from build123d import *

# Parameters (mm, degrees)
Y_KSEKLIK_EKSTR_ZYON1_DEPTH = 100


with BuildPart() as part:
    # Çizim1 → Yükseklik-Ekstrüzyon1 (new body)
    with BuildSketch(Plane.XY.offset(100)):
        with BuildLine():
            Line((6, -28.5), (6, -30))
            Line((6, -30), (26, -30))
            ThreePointArc((26, -30), (28.828427125, -28.828427125), (30, -26))
            Line((30, -26), (30, -6))
            Line((30, -6), (28.5, -6))
            Line((28.5, -6), (28.5, -5))
            Line((28.5, -5), (24, -5))
            Line((24, -5), (24, -10))
            Line((24, -10), (20, -10))
            Line((20, -10), (17, -7))
            Line((17, -7), (17, -0.5))
            Line((17, -0.5), (16.5, 0))
            Line((16.5, 0), (17, 0.5))
            Line((17, 0.5), (17, 7))
            Line((17, 7), (20, 10))
            Line((20, 10), (24, 10))
            Line((24, 10), (24, 5))
            Line((24, 5), (28.5, 5))
            Line((28.5, 5), (28.5, 6))
            Line((28.5, 6), (30, 6))
            Line((30, 6), (30, 26))
            ThreePointArc((30, 26), (28.828427125, 28.828427125), (26, 30))
            Line((26, 30), (6, 30))
            Line((6, 30), (6, 28.5))
            Line((6, 28.5), (5, 28.5))
            Line((5, 28.5), (5, 24))
            Line((5, 24), (10, 24))
            Line((10, 24), (10, 20))
            Line((10, 20), (7, 17))
            Line((7, 17), (0.5, 17))
            Line((0.5, 17), (0, 16.5))
            Line((0, 16.5), (-0.5, 17))
            Line((-0.5, 17), (-7, 17))
            Line((-7, 17), (-10, 20))
            Line((-10, 20), (-10, 24))
            Line((-10, 24), (-5, 24))
            Line((-5, 24), (-5, 28.5))
            Line((-5, 28.5), (-6, 28.5))
            Line((-6, 28.5), (-6, 30))
            Line((-6, 30), (-26, 30))
            ThreePointArc((-26, 30), (-28.828427125, 28.828427125), (-30, 26))
            Line((-30, 26), (-30, 6))
            Line((-30, 6), (-28.5, 6))
            Line((-28.5, 6), (-28.5, 5))
            Line((-28.5, 5), (-24, 5))
            Line((-24, 5), (-24, 10))
            Line((-24, 10), (-20, 10))
            Line((-20, 10), (-17, 7))
            Line((-17, 7), (-17, 0.5))
            Line((-17, 0.5), (-16.5, 0))
            Line((-16.5, 0), (-17, -0.5))
            Line((-17, -0.5), (-17, -7))
            Line((-17, -7), (-20, -10))
            Line((-20, -10), (-24, -10))
            Line((-24, -10), (-24, -5))
            Line((-24, -5), (-28.5, -5))
            Line((-28.5, -5), (-28.5, -6))
            Line((-28.5, -6), (-30, -6))
            Line((-30, -6), (-30, -26))
            ThreePointArc((-30, -26), (-28.828427125, -28.828427125), (-26, -30))
            Line((-26, -30), (-6, -30))
            Line((-6, -30), (-6, -28.5))
            Line((-6, -28.5), (-5, -28.5))
            Line((-5, -28.5), (-5, -24))
            Line((-5, -24), (-10, -24))
            Line((-10, -24), (-10, -20))
            Line((-10, -20), (-7, -17))
            Line((-7, -17), (-0.5, -17))
            Line((-0.5, -17), (0, -16.5))
            Line((0, -16.5), (0.5, -17))
            Line((0.5, -17), (7, -17))
            Line((7, -17), (10, -20))
            Line((10, -20), (10, -24))
            Line((10, -24), (5, -24))
            Line((5, -24), (5, -28.5))
            Line((5, -28.5), (6, -28.5))
        make_face()
        with BuildLine():
            Line((0.832983278, -4.930125652), (1.332773242, -7.88820103))
            ThreePointArc((1.332773242, -7.88820103), (1e-09, -8), (-1.33277324, -7.88820103))
            Line((-1.33277324, -7.88820103), (-0.832983276, -4.930125653))
            ThreePointArc((-0.832983276, -4.930125653), (-1.913417159, -4.619397673), (-2.897117147, -4.075133412))
            Line((-2.897117147, -4.075133412), (-3.476540579, -4.890160098))
            ThreePointArc((-3.476540579, -4.890160098), (-4.242640692, -4.242640704), (-4.890160088, -3.476540593))
            Line((-4.890160088, -3.476540593), (-4.075133404, -2.897117158))
            ThreePointArc((-4.075133404, -2.897117158), (-4.619397678, -1.913417147), (-4.930125659, -0.832983237))
            Line((-4.930125659, -0.832983237), (-7.888201041, -1.332773176))
            ThreePointArc((-7.888201041, -1.332773176), (-8, 3.5e-08), (-7.888201029, 1.332773245))
            Line((-7.888201029, 1.332773245), (-4.930125652, 0.83298328))
            ThreePointArc((-4.930125652, 0.83298328), (-4.619397673, 1.913417161), (-4.075133412, 2.897117148))
            Line((-4.075133412, 2.897117148), (-4.890160097, 3.47654058))
            ThreePointArc((-4.890160097, 3.47654058), (-4.242640703, 4.242640692), (-3.476540592, 4.890160089))
            Line((-3.476540592, 4.890160089), (-2.897117158, 4.075133404))
            ThreePointArc((-2.897117158, 4.075133404), (-1.913417166, 4.619397671), (-0.832983278, 4.930125652))
            Line((-0.832983278, 4.930125652), (-1.332773242, 7.88820103))
            ThreePointArc((-1.332773242, 7.88820103), (-1e-09, 8), (1.33277324, 7.88820103))
            Line((1.33277324, 7.88820103), (0.832983276, 4.930125653))
            ThreePointArc((0.832983276, 4.930125653), (1.913417166, 4.619397671), (2.897117158, 4.075133404))
            Line((2.897117158, 4.075133404), (3.476540592, 4.890160088))
            ThreePointArc((3.476540592, 4.890160088), (4.242640703, 4.242640692), (4.890160098, 3.476540579))
            Line((4.890160098, 3.476540579), (4.075133412, 2.897117147))
            ThreePointArc((4.075133412, 2.897117147), (4.619397681, 1.913417141), (4.930125659, 0.832983237))
            Line((4.930125659, 0.832983237), (7.888201041, 1.332773176))
            ThreePointArc((7.888201041, 1.332773176), (8, -3.5e-08), (7.88820103, -1.332773245))
            Line((7.88820103, -1.332773245), (4.930125652, -0.83298328))
            ThreePointArc((4.930125652, -0.83298328), (4.61939767, -1.913417167), (4.075133404, -2.897117159))
            Line((4.075133404, -2.897117159), (4.890160088, -3.476540593))
            ThreePointArc((4.890160088, -3.476540593), (4.242640698, -4.242640697), (3.476540594, -4.890160088))
            Line((3.476540594, -4.890160088), (2.897117159, -4.075133403))
            ThreePointArc((2.897117159, -4.075133403), (1.913417167, -4.61939767), (0.832983278, -4.930125652))
        make_face(mode=Mode.SUBTRACT)
        with BuildLine():
            Line((12.5, 18.964466094), (12.5, 27.5))
            Line((12.5, 27.5), (27.5, 27.5))
            Line((27.5, 27.5), (27.5, 12.5))
            Line((27.5, 12.5), (18.964466094, 12.5))
            Line((18.964466094, 12.5), (14.5, 8.035533906))
            Line((14.5, 8.035533906), (14.5, 1.250000001))
            Line((14.5, 1.250000001), (9.921567416, 1.250000001))
            ThreePointArc((9.921567416, 1.250000001), (7.071067812, 7.071067812), (1.250000001, 9.921567416))
            Line((1.250000001, 9.921567416), (1.250000001, 14.5))
            Line((1.250000001, 14.5), (8.035533906, 14.5))
            Line((8.035533906, 14.5), (12.5, 18.964466094))
        make_face(mode=Mode.SUBTRACT)
        with BuildLine():
            Line((18.964466094, -12.5), (27.5, -12.5))
            Line((27.5, -12.5), (27.5, -27.5))
            Line((27.5, -27.5), (12.5, -27.5))
            Line((12.5, -27.5), (12.5, -18.964466094))
            Line((12.5, -18.964466094), (8.035533906, -14.5))
            Line((8.035533906, -14.5), (1.250000001, -14.5))
            Line((1.250000001, -14.5), (1.250000001, -9.921567416))
            ThreePointArc((1.250000001, -9.921567416), (7.071067812, -7.071067812), (9.921567416, -1.250000001))
            Line((9.921567416, -1.250000001), (14.5, -1.250000001))
            Line((14.5, -1.250000001), (14.5, -8.035533906))
            Line((14.5, -8.035533906), (18.964466094, -12.5))
        make_face(mode=Mode.SUBTRACT)
        with BuildLine():
            Line((-12.5, -18.964466094), (-12.5, -27.5))
            Line((-12.5, -27.5), (-27.5, -27.5))
            Line((-27.5, -27.5), (-27.5, -12.5))
            Line((-27.5, -12.5), (-18.964466094, -12.5))
            Line((-18.964466094, -12.5), (-14.5, -8.035533906))
            Line((-14.5, -8.035533906), (-14.5, -1.250000001))
            Line((-14.5, -1.250000001), (-9.921567416, -1.250000001))
            ThreePointArc((-9.921567416, -1.250000001), (-7.071067812, -7.071067812), (-1.250000001, -9.921567416))
            Line((-1.250000001, -9.921567416), (-1.250000001, -14.5))
            Line((-1.250000001, -14.5), (-8.035533906, -14.5))
            Line((-8.035533906, -14.5), (-12.5, -18.964466094))
        make_face(mode=Mode.SUBTRACT)
        with BuildLine():
            Line((-18.964466094, 12.5), (-27.5, 12.5))
            Line((-27.5, 12.5), (-27.5, 27.5))
            Line((-27.5, 27.5), (-12.5, 27.5))
            Line((-12.5, 27.5), (-12.5, 18.964466094))
            Line((-12.5, 18.964466094), (-8.035533906, 14.5))
            Line((-8.035533906, 14.5), (-1.250000001, 14.5))
            Line((-1.250000001, 14.5), (-1.250000001, 9.921567416))
            ThreePointArc((-1.250000001, 9.921567416), (-7.071067812, 7.071067812), (-9.921567416, 1.250000001))
            Line((-9.921567416, 1.250000001), (-14.5, 1.250000001))
            Line((-14.5, 1.250000001), (-14.5, 8.035533906))
            Line((-14.5, 8.035533906), (-18.964466094, 12.5))
        make_face(mode=Mode.SUBTRACT)
    extrude(amount=-Y_KSEKLIK_EKSTR_ZYON1_DEPTH)


solid = part.part
CAD build for the part. Positions are in the model's coordinates, mm. A direction names the side the tool comes from. Give positions to 0.01 mm unless a question says otherwise; leave off trailing zeros. Write each loop counter-clockwise with the first axis right and the second up, starting at its lowest first coordinate (ties: lowest second). Pieces come first, ordered by that corner, then holes. Notation, with made-up numbers: (17, -32) - (27, -32) arc R12 ccw to (27, -25) - close; hole circle Ø3 at (-32.75, 0.25). An arc over 180 degrees is marked (long way). Answer as CSV lines item,"result".
Q1. Drill centre lines: line 1 (X direction, y = -21.5, z = 12); line 2 (X direction, y = -25, z = 9). Where is each one in solid material? Low to high. Write a range as from..to.
Result set:
line 1,"-30..-27.5, -12.5..-10, 10..12.5, 27.5..30"
line 2,"-30..-27.5, -12.5..-5, 5..12.5, 27.5..30"
Q2. Band-saw the part on C-C (z = 26.5). State how many separate pieces and enclosed holes the cut face has, and give its area (3 significant figures).
Result set:
separate pieces,"1"
enclosed holes,"5"
area,"1,250 mm²"
Q3. Band-saw the part on A-A (x = 21.5). Give the cut face in (y, z), and give its area (3 significant figures).
Result set:
outline,"(-30, 0) - (-27.5, 0) - (-27.5, 100) - (-30, 100) - close; (-12.5, 0) - (-10, 0) - (-10, 100) - (-12.5, 100) - close; (10, 0) - (12.5, 0) - (12.5, 100) - (10, 100) - close; (27.5, 0) - (30, 0) - (30, 100) - (27.5, 100) - close"
area,"1,000 mm²"
Q4. Pull direction X, two halves, no side cores. Call faces 1 (the face through (30, -16, 51)), 2 (the face through (-16, -30, 51)), 3 (the face through (0, 8, 51)): released by +X, released by -X, zero draft, split by the parting line, or undercut.
Result set:
face 1,"released by +X"
face 2,"zero draft"
face 3,"undercut"
Q5. Flat gauge pins, fed straight in: pin 1 Ø1.5 at (y, z) = (-3.5, 49.5) entering from +X; pin 2 Ø3 at (x, y) = (-16, 13) entering from -Z. Where does each tip first touch, or does it go through?
Result set:
pin 1,"x = 17"
pin 2,"through"
Q6. 3-axis set-ups, long thin cutter, end or side, ignore diameter. For faces 4 (the face through (-1.899, -4.625, 50.7)), 5 (the face through (26, 5, 51)): which of +Z, -Z, +X, -X, +Y, -Y reach the whole face in a straight line?
Result set:
face 4,"+Z, -Z"
face 5,"+Z, -Z, +X"
